```python
from build123d import *

# Parameters (mm, degrees)
F0_W     = 254
F0_H     = 152.4
F1_DEPTH = 228.6
F2_DEPTH = 6.35
F4_DEPTH = 25.4


with BuildPart() as f1:
    # F0 (on Top) → F1 (new body)
    with BuildSketch(Plane.XY):
        Polygon((257.823838, 32.772094), (-21.576162, 32.772094), (-21.576162, -94.227906), (-250.176162, -94.227906), (-250.176162, -145.027906), (257.823838, -145.027906), align=None)
        with Locations((118.123838, -56.127906)):
            Rectangle(F0_W, F0_H, mode=Mode.SUBTRACT)
        with Locations((118.123838, -56.127906)):
            Rectangle(F0_W, F0_H)
    extrude(amount=-F1_DEPTH)

    # F0 (on Top) → F2 (cut)
    with BuildSketch(Plane.XY):
        with Locations((118.123838, -56.127906)):
            Rectangle(F0_W, F0_H)
    extrude(amount=-F2_DEPTH, mode=Mode.SUBTRACT)

    # F3 (on face) → F4 (cut)
    with BuildSketch(Plane(origin=(0, -94.227906, 0), x_dir=(-1, 0, 0), z_dir=(0, 1, 0))):
        with BuildLine():
            ThreePointArc((237.476162, -114.3), (207.71821, -42.457951), (135.876162, -12.7))
            ThreePointArc((135.876162, -12.7), (64.034113, -186.142049), (237.476162, -114.3))
        make_face()
        with BuildLine():
            ThreePointArc((234.301162, -114.3), (66.279177, -183.896985), (135.876162, -15.875))
            ThreePointArc((135.876162, -15.875), (205.473146, -44.703015), (234.301162, -114.3))
        make_face(mode=Mode.SUBTRACT)
    extrude(amount=-F4_DEPTH, mode=Mode.SUBTRACT)


solid = f1.part
```
Input: part model. Units: mm. Frame: model coordinates. A direction names the side the tool comes from. Round coordinates to 2 decimals unless told otherwise and drop trailing zeros. Loops run counter-clockwise (first coordinate to the right, second up) from the corner with the lowest first, then second, coordinate; pieces in that order, holes last. Notation, with made-up numbers: (30.25, -12.5) -> (39.25, -12.5) arc R10 ccw to (39.25, -6.5) -> close; hole circle Ø6 at (54.5, 9). An arc over 180 degrees is marked (long way). Write each question's results on one line, items separated by ' | '.
1. Section B-B (x = 162). Return loops of the section in (y, z), and give its area (3 significant figures).
Geometry results:
outline: (-145.03, -228.6) -> (32.77, -228.6) -> (32.77, 0) -> (20.07, 0) -> (20.07, -6.35) -> (-132.33, -6.35) -> (-132.33, 0) -> (-145.03, 0) -> close | area: 39,700 mm2
2. Section D-D (z = -140). Return loops of the section in (x, y), and give its area (3 significant figures).
Geometry results:
outline: (-250.18, -145.03) -> (257.82, -145.03) -> (257.82, 32.77) -> (-21.58, 32.77) -> (-21.58, -94.23) -> (-37.58, -94.23) -> (-37.58, -119.63) -> (-40.87, -119.63) -> (-40.87, -94.23) -> (-230.89, -94.23) -> (-230.89, -119.63) -> (-234.17, -119.63) -> (-234.17, -94.23) -> (-250.18, -94.23) -> close | area: 61,100 mm2
3. Ray query, line 1 (X direction, y = -101.5, z = -77.5); line 2 (X direction, y = -102.5, z = -67); line 3 (Y direction, x = -50.5, z = -197). Return the intervals inside material, ascending. Write a range as from..to.
Geometry results:
line 1: -250.18..-230.58, -227.16..-44.59, -41.17..257.82 | line 2: -250.18..-225.79, -222.19..-49.56, -45.96..257.82 | line 3: -145.03..-94.23
4. Section A-A (y = 2.5). Return loops of the section in (x, z).
Geometry results:
outline: (-21.58, -228.6) -> (257.82, -228.6) -> (257.82, 0) -> (245.12, 0) -> (245.12, -6.35) -> (-8.88, -6.35) -> (-8.88, 0) -> (-21.58, 0) -> close
5. First-contact query: P1, Ø1.5, axis at x = 32, y = -25, coming from the +Z side; P2, Ø6, axis at x = -166, z = -102, coming from the +Y side; P3, Ø2, axis at x = -13, y = -122, coming from the +Z side; P4, Ø3, axis at y = -19.5, z = -4.5, coming from the -X side. Flat tips, straight axial feed; report the tip coordinate or a pass-through.
Geometry results:
P1: z = -6.35 | P2: y = -94.23 | P3: z = 0 | P4: x = -21.58
6. Section C-C (z = -77.5). Return loops of the section in (x, y).
Geometry results:
outline: (-250.18, -145.03) -> (257.82, -145.03) -> (257.82, 32.77) -> (-21.58, 32.77) -> (-21.58, -94.23) -> (-41.17, -94.23) -> (-41.17, -119.63) -> (-44.59, -119.63) -> (-44.59, -94.23) -> (-227.16, -94.23) -> (-227.16, -119.63) -> (-230.58, -119.63) -> (-230.58, -94.23) -> (-250.18, -94.23) -> close
7. Mould query, pull axis X, two halves, no side actions, for faces 1 (the face through (-134, -94.228, -113)), 2 (the face through (116, -55, -6.35)), 3 (the face through (257.824, -57, -113)). Classes: +X half, -X half, draft (parallel to the pull), parting line (faces both ways), or undercut.
Geometry results:
face 1: draft | face 2: undercut | face 3: +X half
8. Set-up query: faces 4 (the face through (-83, -119.628, -31)), 5 (the face through (120, 32.772, -113)), 6 (the face through (-33, -94.228, -113)). Return all of +Z, -Z, +X, -X, +Y, -Y with unobstructed straight access to the full face (end or side cutting, diameter ignored); none if empty.
Geometry results:
face 4: +Y | face 5: +Z, -Z, +X, -X, +Y | face 6: +Z, -Z, -X, +Y
